Check sheet for the modelled part. Datum: model origin and axes. Units: mm. A direction names the side the tool comes from. Give positions to 0.01 mm unless a question says otherwise; leave off trailing zeros. Order: outer loops, then holes, each group sorted by start corner. A loop starts at its lowest first (then second) coordinate and runs counter-clockwise, first axis right, second up. Notation, with made-up numbers: (44, 68.25) - (65, 68.25) arc R30 ccw to (65, 105.25) - close; hole circle Ø4 at (32, 43.5). An arc over 180 degrees is marked (long way). Answer in a Markdown table with one row per item.
from build123d import *

# Parameters (mm, degrees)
SKETCH_2_W              = 71
SKETCH_2_H              = 55
EXTRUDE_1_DEPTH         = 2
HOLE_WIZARD_6_2_6_2_1_D = 6.2
FILLET_1_R              = 5


with BuildPart() as part:
    # 草图1 → 旋转1 (revolve)
    with BuildSketch(Plane(origin=(0, 0, 0), x_dir=(-1, 0, 0), z_dir=(0, 0, -1)), mode=Mode.PRIVATE) as revolve_1_sk:
        with BuildLine():
            Line((-17, -2), (0, -2))
            Line((0, -2), (0, 0))
            Line((0, 0), (-17, 0))
            ThreePointArc((-17, 0), (-18.414213562, 0.585786438), (-19, 2))
            Line((-19, 2), (-21, 2))
            ThreePointArc((-21, 2), (-19.828427125, -0.828427125), (-17, -2))
        make_face()
    revolve(revolve_1_sk.sketch.rotate(Axis((0, -2.005, 0), (0, 1, 0)), 270), axis=Axis((0, -2.005, 0), (0, 1, 0)))

    # 草图2 → 凸台-拉伸1 (add)
    with BuildSketch(Plane(origin=(0, -2, 0), x_dir=(1, 0, 0), z_dir=(0, 1, 0))):
        Rectangle(SKETCH_2_W, SKETCH_2_H)
    extrude(amount=-EXTRUDE_1_DEPTH)

    # 草图3 → 旋转2 (revolve)
    with BuildSketch(Plane(origin=(0, 0, 0), x_dir=(-1, 0, 0), z_dir=(0, 0, -1)), mode=Mode.PRIVATE) as revolve_2_sk:
        Polygon((-5, 0), (0, 0), (0, 6), (-9, 6), (-9, 4), (-5, 4), align=None)
    revolve(revolve_2_sk.sketch.rotate(Axis((0, 0, 0), (0, 1, 0)), 270), axis=Axis((0, 0, 0), (0, 1, 0)))

    # Ø6.2 (6.2) 直径孔1 (through all)
    with Locations(Plane(origin=(0, -2, 0), x_dir=(1, 0, 0), z_dir=(0, 1, 0))):
        with Locations((-27.5, 18), (-27.5, -18), (27.5, -18), (27.5, 18)):
            Hole(HOLE_WIZARD_6_2_6_2_1_D / 2)

    # 圆角1
    fillet_1_edges = [part.edges().sort_by_distance(p)[0] for p in [
        (35.5, -3, -27.5),
        (35.5, -3, 27.5),
        (-35.5, -3, 27.5),
        (-35.5, -3, -27.5),
    ]]
    fillet(fillet_1_edges, radius=FILLET_1_R)


solid = part.part
(1) Cross-section at D-D, the plane z = 18. Give the number of separate pieces and of enclosed holes in the cut face, then the cut area to 3 significant figures.
Geometry says:
| item | result |
|---|---|
| separate pieces | 4 |
| enclosed holes | 0 |
| area | 170 mm² |
(2) Cross-section at C-C, the plane y = 5. Record the cut outline in (x, z).
Geometry says:
| item | result |
|---|---|
| outline | circle Ø18 at (0, 0) |
(3) Mould release check, pull along X, two halves, no side actions. Record for faces 1 (the flat face through (35.5, -3, 0)), 2 (the cylindrical face through (2.703, 4.986, 8.584)), 3 (the cylindrical face through (-25.04, -3.014, -16.114)): pulls with the +X half, pulls with the -X half, needs draft (parallel to the pull), parting line crosses it, or undercut.
Geometry says:
| item | result |
|---|---|
| face 1 | pulls with the +X half |
| face 2 | parting line crosses it |
| face 3 | undercut |
(4) Thickness scan on L1, parallel to X at y = -3.25, z = -18; L2, parallel to Z at x = 27.5, y = -3.1; L3, parallel to Y at x = -5.5, z = -8.5. Record the ranges inside material, lowest first.
Geometry says:
| item | result |
|---|---|
| L1 | -35.5 to -30.6, -24.4 to 24.4, 30.6 to 35.5 |
| L2 | -27.5 to -21.1, -14.9 to 14.9, 21.1 to 27.5 |
| L3 | -4 to 0 |
(5) Gauge pin test, flat ends, axial feed: P1, Ø5.5, axis at x = 27.5, z = -18, coming from the +Y side; P2, Ø2, axis at x = 14, y = 1.5, coming from the +Z side; P3, Ø16.5, axis at x = 12.5, z = 12.5, coming from the +Y side; P4, Ø5, axis at x = -8, y = 3.5, coming from the +Z side. Record the tip position at first contact, or that the pin passes through.
Geometry says:
| item | result |
|---|---|
| P1 | through |
| P2 | z = 16.46 |
| P3 | y = 2 |
| P4 | z = 20.12 |
(6) Access from +Z, -Z, +X, -X, +Y, -Y to the whole of each face (thin tool, end or side, straight path). Record for faces 4 (the flat face through (-4, 0, -4)), 5 (the flat face through (0, -4, 0)).
Geometry says:
| item | result |
|---|---|
| face 4 | none |
| face 5 | +Z, -Z, +X, -X, -Y |
(7) Cross-section at A-A, the plane x = 27.5. Record the cut outline in (y, z).
Geometry says:
| item | result |
|---|---|
| outline | (-4, -27.5) - (-2, -27.5) - (-2, -21.1) - (-4, -21.1) - close; (-4, -14.9) - (-2, -14.9) - (-2, 14.9) - (-4, 14.9) - close; (-4, 21.1) - (-2, 21.1) - (-2, 27.5) - (-4, 27.5) - close |
(8) Cross-section at B-B, the plane z = 0. Record the cut outline in (x, y).
Geometry says:
| item | result |
|---|---|
| outline | (-35.5, -4) - (35.5, -4) - (35.5, -2) - (17, -2) arc R4 ccw to (21, 2) - (19, 2) arc R2 cw to (17, 0) - (5, 0) - (5, 4) - (9, 4) - (9, 6) - (-9, 6) - (-9, 4) - (-5, 4) - (-5, 0) - (-17, 0) arc R2 cw to (-19, 2) - (-21, 2) arc R4 ccw to (-17, -2) - (-35.5, -2) - close |
